Here's how the part is built. I have some questions about the finished solid (model axes, mm). Round coordinates to 2 decimals unless told otherwise and drop trailing zeros. Write each loop counter-clockwise with the first axis right and the second up, starting at its lowest first coordinate (ties: lowest second). Pieces come first, ordered by that corner, then holes. Notation, with made-up numbers: (-34.75, 24.25) - (12.25, 24.25) arc R23 cw to (12.25, 61.25) - close; hole circle Ø1 at (-8, 78.5). An arc over 180 degrees is marked (long way). One line per item, written item: value. Start each with the question number.
Item 1: If I drill on line 1 (Y direction, x = -10, z = 4); line 2 (X direction, y = -4, z = -3); line 3 (Y direction, x = -63, z = -2), over which ranges is the centre line in solid material (lowest first)?
Item 2: For P1, Ø12, axis at y = 18.5, z = -3, coming from the +X side; P2, Ø3, axis at y = -0.5, z = -6, coming from the +X side; P3, Ø10, axis at y = 7, z = 3, coming from the +X side; P4, Ø12, axis at x = -66, z = -4, coming from the -Y side, each with a flat end and sliding along its axis, tell me the tip position at first contact or that it passes through.
Item 3: Imagine slicing it at B-B, the plane z = 2.5. Please give me the cut outline in (x, y), then the cut area to 3 significant figures.
Item 4: Imagine slicing it at A-A, the plane y = 0. Please give me the cut outline in (x, z) (3 decimals).
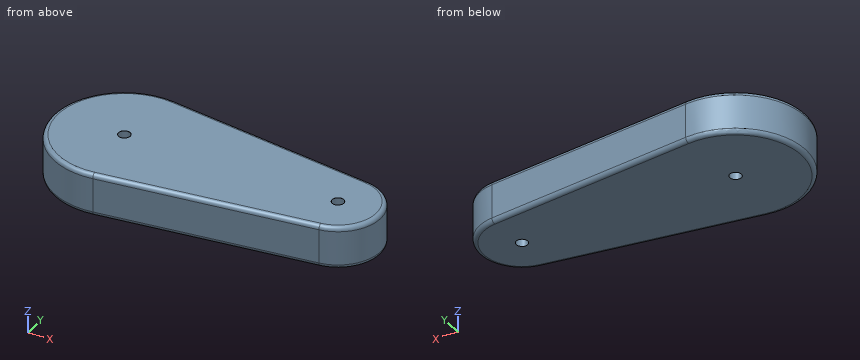
```python
from build123d import *

# Parameters (mm, degrees)
BRAS_DEPTH              = 10
PER_AGE_M51_D           = 5.5
PER_AGE_M51_CSINK_D     = 5.55
PER_AGE_M51_CSINK_ANGLE = 90
CONG_1_R                = 2


with BuildPart() as part:
    # Profil Bras → Bras (new, symmetric)
    with BuildSketch(Plane.XY):
        with BuildLine():
            Line((-46.102514264, 32.881516449), (53.041971873, 19.828897227))
            ThreePointArc((53.041971873, 19.828897227), (70.431448029, 0), (53.041971873, -19.828897227))
            Line((53.041971873, -19.828897227), (-46.102514264, -32.881516449))
            ThreePointArc((-46.102514264, -32.881516449), (-83.596697788, 0), (-46.102514264, 32.881516449))
        make_face()
    extrude(amount=BRAS_DEPTH, both=True)

    # Perçage M51 (through all)
    with Locations(Plane.XY.offset(10)):
        with Locations((-50.431448029, 0), (50.431448029, 0)):
            CounterSinkHole(PER_AGE_M51_D / 2, PER_AGE_M51_CSINK_D / 2, counter_sink_angle=PER_AGE_M51_CSINK_ANGLE)

    # Congé1
    cong_1_edges = [part.edges().sort_by_distance(p)[0] for p in [
        (70.431448029, 0, 10),
        (3.469728805, 26.355206838, 10),
        (-83.596697788, 0, 10),
        (3.469728805, 26.355206838, -10),
        (70.431448029, 0, -10),
        (3.469728805, -26.355206838, -10),
        (-83.596697788, 0, -10),
        (3.469728805, -26.355206838, 10),
    ]]
    fillet(cong_1_edges, radius=CONG_1_R)


solid = part.part
```
Values follow:
1. line 1: y = -28.13 to 28.13
1. line 2: x = -83.35 to 70.03
1. line 3: y = -30.69 to 30.69
2. P1: stops at x = 66.04
2. P2: stops at x = 70.43
2. P3: stops at x = 70.33
2. P4: stops at y = -31.75
3. outline: (-46.1, -32.88) - (53.04, -19.83) arc R20 ccw to (53.04, 19.83) - (-46.1, 32.88) arc R33.17 ccw (long way) to start; hole circle Ø5.5 at (-50.43, 0); hole circle Ø5.5 at (50.43, 0)
3. area: 7,720 mm^2
4. outline: (-83.597, -8) arc R2 ccw to (-81.597, -10) - (-53.181, -10) - (-53.181, 9.975) - (-53.206, 10) - (-81.597, 10) arc R2 ccw to (-83.597, 8) - close; (-47.681, -10) - (47.681, -10) - (47.681, 9.975) - (47.656, 10) - (-47.656, 10) - (-47.681, 9.975) - close; (53.181, -10) - (68.431, -10) arc R2 ccw to (70.431, -8) - (70.431, 8) arc R2 ccw to (68.431, 10) - (53.206, 10) - (53.181, 9.975) - close
